```python
from build123d import *

# Parameters (mm, degrees)
F0_W      = 345
F0_H      = 223.5
F1_DEPTH  = 2.75
F2_W      = 336.5
F2_H      = 212.5
F3_DEPTH  = 0.5
F5_DEPTH  = 1
F7_DEPTH  = 1
F8_R      = 1.5
F8_R_2    = 2
F9_DEPTH  = 1
F10_R     = 1.5
F10_R_2   = 2
F11_DEPTH = 1
F12_W     = 35.267069459
F12_H     = 5.5
F13_DEPTH = 1
F14_W     = 17.2233697499
F14_H     = 8.9206725706
F14_R     = 2
F15_DEPTH = 1
F16_R     = 2.1707267793
F17_DEPTH = 50
F18_W     = 43.8106725812
F18_H     = 5.5
F19_DEPTH = 1
F20_W     = 17.3314685191
F20_H     = 8.8958692735
F20_R     = 2
F21_DEPTH = 1
F22_R     = 2.2669992326
F23_DEPTH = 50


with BuildPart() as f1:
    # F0 (on Top) → F1 (new body, symmetric)
    with BuildSketch(Plane.XY):
        Rectangle(F0_W, F0_H)
    extrude(amount=F1_DEPTH, both=True)

    # F2 (on face) → F3 (cut)
    with BuildSketch(Plane.XY.offset(2.75)):
        with Locations((0.75, 0)):
            Rectangle(F2_W, F2_H)
    extrude(amount=-F3_DEPTH, mode=Mode.SUBTRACT)

    # F4 (on face) → F5 (join)
    with BuildSketch(Plane(origin=(-172.5, 0, 0), x_dir=(0, -1, 0), z_dir=(-1, 0, 0))):
        Polygon((-111.75, 2.75), (-124.75, 2.75), (-124.75, -2.75), (-111.75, -2.75), (111.75, -2.75), (130.75, -2.75), (130.75, 2.75), (111.75, 2.75), align=None)
    extrude(amount=F5_DEPTH)

    # F6 (on face) → F7 (join)
    with BuildSketch(Plane.YZ.offset(172.5)):
        Polygon((124.75, 2.75), (111.75, 2.75), (-111.75, 2.75), (-130.75, 2.75), (-130.75, -2.75), (-111.75, -2.75), (111.75, -2.75), (124.75, -2.75), align=None)
    extrude(amount=F7_DEPTH)

    # F8 (on face) → F9 (join)
    with BuildSketch(Plane(origin=(0, 0, -2.75), x_dir=(1, 0, 0), z_dir=(0, 0, -1))):
        Polygon((-172.5, -117.75), (-172.5, -124.75), (-172.5, -129.75), (-165, -129.75), (-165, -117.75), align=None)
        with Locations((-168.75, -127.25)):
            Circle(F8_R, mode=Mode.SUBTRACT)
        with Locations((-168.75, -121.75)):
            Circle(F8_R_2, mode=Mode.SUBTRACT)
    extrude(amount=-F9_DEPTH)

    # F10 (on face) → F11 (join)
    with BuildSketch(Plane(origin=(0, 0, -2.75), x_dir=(1, 0, 0), z_dir=(0, 0, -1))):
        Polygon((165, -117.75), (165, -129.75), (172.5, -129.75), (172.5, -124.75), (172.5, -117.75), align=None)
        with Locations((168.75, -127.25)):
            Circle(F10_R, mode=Mode.SUBTRACT)
        with Locations((168.75, -121.75)):
            Circle(F10_R_2, mode=Mode.SUBTRACT)
    extrude(amount=-F11_DEPTH)

    # F12 (on face) → F13 (join)
    with BuildSketch(Plane(origin=(-173.5, 0, 0), x_dir=(0, -1, 0), z_dir=(-1, 0, 0))):
        with Locations((113.1164652705, 0)):
            Rectangle(F12_W, F12_H)
    extrude(amount=F13_DEPTH)

    # F14 (on face) → F15 (join)
    with BuildSketch(Plane(origin=(0, 0, -2.75), x_dir=(1, 0, 0), z_dir=(0, 0, -1))):
        with Locations((-163.8883151251, 119.3223506039)):
            Rectangle(F14_W, F14_H)
        with Locations((-169.4210810497, 117.5438189247)):
            Circle(F14_R, mode=Mode.SUBTRACT)
        with Locations((-163.8866538361, 117.5438189247)):
            Circle(F14_R, mode=Mode.SUBTRACT)
        with Locations((-158.6872041225, 121.0242956877)):
            Circle(F14_R, mode=Mode.SUBTRACT)
    extrude(amount=-F15_DEPTH)

    # F16 (on face) → F17 (join)
    with BuildSketch(Plane.YZ.offset(-172.5)):
        with Locations((-127.9121488333, 0)):
            Circle(F16_R)
    extrude(amount=F17_DEPTH)

    # F18 (on face) → F19 (join)
    with BuildSketch(Plane.YZ.offset(173.5)):
        with Locations((-108.8446637094, 0)):
            Rectangle(F18_W, F18_H)
    extrude(amount=F19_DEPTH)

    # F20 (on face) → F21 (join)
    with BuildSketch(Plane(origin=(0, 0, -2.75), x_dir=(1, 0, 0), z_dir=(0, 0, -1))):
        with Locations((163.8342657404, 117.9346791002)):
            Rectangle(F20_W, F20_H)
        with Locations((163.4575277567, 116.1992102861)):
            Circle(F20_R, mode=Mode.SUBTRACT)
        with Locations((158.4874242544, 119.7936609387)):
            Circle(F20_R, mode=Mode.SUBTRACT)
        with Locations((169.3595200777, 116.1992102861)):
            Circle(F20_R, mode=Mode.SUBTRACT)
    extrude(amount=-F21_DEPTH)

    # F22 (on face) → F23 (join)
    with BuildSketch(Plane(origin=(172.5, 0, 0), x_dir=(0, -1, 0), z_dir=(-1, 0, 0))):
        with Locations((126.5941113234, 0)):
            Circle(F22_R)
    extrude(amount=F23_DEPTH)


solid = f1.part
```
Source: CAD feature listing. Evaluate the final solid. Frame: model axes, mm. A direction names the side the tool comes from. Give positions to 0.01 mm unless a question says otherwise; leave off trailing zeros. Write each loop counter-clockwise with the first axis right and the second up, starting at its lowest first coordinate (ties: lowest second). Pieces come first, ordered by that corner, then holes. Notation, with made-up numbers: (78, 56.25) - (104, 56.25) arc R18 cw to (104, 81.25) - close; hole circle Ø2 at (-17, 22.25). An arc over 180 degrees is marked (long way). One line per item, written item: value. Start each with the question number.
Q1. Section query A-A, the plane x = 138. Return the cut outline in (y, z), then the cut area to 3 significant figures.
Q2. Draft query along Y for faces 1 (the face through (-2, 1, 2.25)), 2 (the face through (-164, -120, -1.75)), 3 (the face through (-168, 124, -1.75)). Return one class per face: +Y half, -Y half, draft (parallel to the pull), parting line (faces both ways), or undercut.
Q3. Set-up query: faces 4 (the face through (164, -119, -1.75)), 5 (the face through (-53, -108, 2.75)), 6 (the face through (170, 124, -1.75)). Return all of +Z, -Z, +X, -X, +Y, -Y with unobstructed straight access to the full face (end or side cutting, diameter ignored); none if empty.
Q4. Section query C-C, the plane z = 0. Return the cut outline in (x, y), then the cut area to 3 significant figures.
Q5. Section query B-B, the plane y = 85. Return the cut outline in (x, z), then the cut area to 3 significant figures.
Q6. Material intervals for probe 1 along X at (y, z) = (121.75, -1.95); probe 2 along X at (y, z) = (127.25, -2.3); probe 3 along X at (y, z) = (53.5, 2.45), sorted ascending. Write a range as from..to.
Q7. Section query D-D, the plane x = -133.5. Return the cut outline in (y, z), then the cut area to 3 significant figures.
Q8. First-contact query: pin 1 Ø1.5 at (x, z) = (-103.5, -0.5) entering from +Y; pin 2 Ø2.5 at (x, y) = (168.75, 127.25) entering from -Z; pin 3 Ø0.5 at (x, z) = (-173, -1) entering from +Y; pin 4 Ø4 at (x, y) = (170.5, 126) entering from +Z. Flat tips, straight axial feed; report the tip coordinate or a pass-through.
Answer:
1. outline: circle Ø4.53 at (-126.59, 0); (-111.75, -2.75) - (111.75, -2.75) - (111.75, 2.75) - (106.25, 2.75) - (106.25, 2.25) - (-106.25, 2.25) - (-106.25, 2.75) - (-111.75, 2.75) - close
1. area: 1,140 mm2
2. face 1: undercut
2. face 2: undercut
2. face 3: draft
3. face 4: +Z
3. face 5: +Z, +X, -X, +Y, -Y
3. face 6: +Z, +Y
4. outline: (-174.5, -130.75) - (-172.5, -130.75) - (-172.5, -130.08) - (-122.5, -130.08) - (-122.5, -125.74) - (-172.5, -125.74) - (-172.5, -111.75) - (172.5, -111.75) - (172.5, -124.33) - (122.5, -124.33) - (122.5, -128.86) - (172.5, -128.86) - (172.5, -130.75) - (174.5, -130.75) - (174.5, -86.94) - (173.5, -86.94) - (173.5, 124.75) - (172.5, 124.75) - (172.5, 111.75) - (-172.5, 111.75) - (-172.5, 124.75) - (-173.5, 124.75) - (-173.5, -95.48) - (-174.5, -95.48) - close
4. area: 78,100 mm2
5. outline: (-173.5, -2.75) - (173.5, -2.75) - (173.5, 2.75) - (169, 2.75) - (169, 2.25) - (-167.5, 2.25) - (-167.5, 2.75) - (-173.5, 2.75) - close
5. area: 1,740 mm2
6. probe 1: x = -173.5..-170.75, -166.75..-165, 165..166.75, 170.75..173.5
6. probe 2: x = -172.5..-170.25, -167.25..-165, 165..167.25, 170.25..172.5
6. probe 3: x = -173.5..-167.5, 169..173.5
7. outline: circle Ø4.34 at (-127.91, 0); (-111.75, -2.75) - (111.75, -2.75) - (111.75, 2.75) - (106.25, 2.75) - (106.25, 2.25) - (-106.25, 2.25) - (-106.25, 2.75) - (-111.75, 2.75) - close
7. area: 1,140 mm2
8. pin 1: stops at y = 111.75
8. pin 2: passes through
8. pin 3: stops at y = 124.75
8. pin 4: stops at z = -1.75
